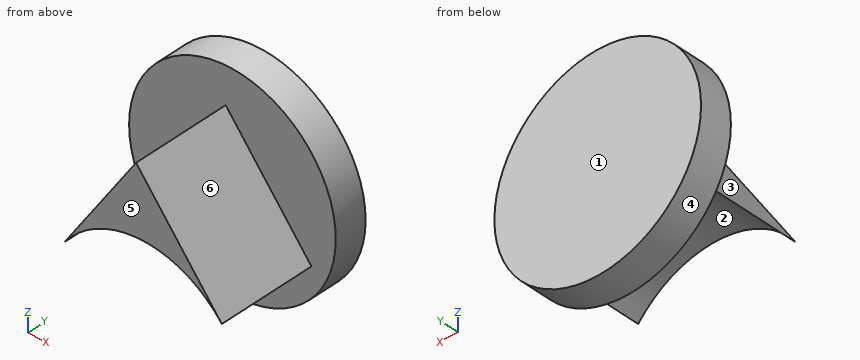
from build123d import *

# Parameters (mm, degrees)
F0_R     = 81.624409
F1_DEPTH = 25.4
F3_DEPTH = 76.2


with BuildPart() as f1:
    # F0 (on Front) → F1 (new body)
    with BuildSketch(Plane.XZ):
        with Locations((-32.545008, 13.374658)):
            Circle(F0_R)
    extrude(amount=F1_DEPTH)

    # F2 (on face) → F3 (join)
    with BuildSketch(Plane.XZ.offset(25.4)):
        with BuildLine():
            Line((-37.894875, 66.024758), (-94.514281, -20.018902))
            ThreePointArc((-94.514281, -20.018902), (-33.306834, 12.514138), (29.870085, -16.006503))
            Line((29.870085, -16.006503), (-37.894875, 66.024758))
        make_face()
    extrude(amount=F3_DEPTH)


solid = f1.part
Input: part model. Units: mm. Frame: model coordinates. Face numbers are marked on the shaded views. A direction names the side the tool comes from. Coordinates: 2 decimals unless noted, no trailing zeros. Loops run counter-clockwise (first coordinate to the right, second up) from the corner with the lowest first, then second, coordinate; pieces in that order, holes last. Notation, with made-up numbers: (9.25, 30.25) - (42.25, 30.25) arc R15 cw to (42.25, 41.25) - close; hole circle Ø10 at (78.25, 68). An arc over 180 degrees is marked (long way). Answer in a Markdown table with one row per item. Add a question column.
Item 1: Section query B-B on z = 10. Return the cut outline in (x, y), then the cut area to 3 significant figures.
Item 2: Contact query for flat-ended pins moving along their axis: P1, Ø8, axis at y = -59, z = -15.5, coming from the -X side; P2, Ø1.5, axis at y = -18, z = 47, coming from the +X side; P3, Ø3, axis at x = 17, z = 39, coming from the +Y side; P4, Ø2, axis at y = -87.5, z = 34.5, coming from the +X side. Output: stop coordinate, or through.
Item 3: Section query A-A on x = -70. Return the cut outline in (y, z).
Item 4: Access query for the marked faces 5 and 6. Directions: +Z, -Z, +X, -X, +Y, -Y. A direction counts if a zero-diameter tool reaches every point of the face in a straight line with its end or side. Return the directions, or none.
Item 5: Line query: line 1 along Y through (x, z) = (-2.5, 86); line 2 along Z through (x, y) = (-31, -12.5); line 3 along X through (y, z) = (-20, 14.5). Output: solid intervals per line, ascending. Write a range as [from, to].
Item 6: Mould query, pull axis X, two halves, no side actions, for the marked faces 1, 2, 3 and 4. Classes: released by +X, released by -X, zero draft, split by the parting line, or undercut.
Item 7: Section query D-D on x = 6.5. Return the cut outline in (y, z).
Item 8: Section query C-C on y = -64.5. Return the cut outline in (x, z), then the cut area to 3 significant figures.
Recorded:
| question | item | result |
|---|---|---|
| 1 | outline | (-114.1, -25.4) - (-74.76, -25.4) - (-74.76, -101.6) - (-50.66, -101.6) - (-50.66, -25.4) - (-10.89, -25.4) - (-10.89, -101.6) - (8.39, -101.6) - (8.39, -25.4) - (49.01, -25.4) - (49.01, 0) - (-114.1, 0) - close |
| 1 | area | 7,450 mm^2 |
| 2 | P1 | x = -94.17 |
| 2 | P2 | x = 42.17 |
| 2 | P3 | y = 0 |
| 2 | P4 | x = -11.03 |
| 3 | outline | (-101.6, 2.07) - (-25.4, 2.07) - (-25.4, -59.15) - (0, -59.15) - (0, 85.9) - (-25.4, 85.9) - (-25.4, 17.24) - (-101.6, 17.24) - close |
| 4 | face 5 | +Z, -Z, +X, -X, -Y |
| 4 | face 6 | +Z, +X, -Y |
| 5 | line 1 | [-25.4, 0] |
| 5 | line 2 | [-68.24, 94.98] |
| 5 | line 3 | [-114.16, 49.07] |
| 6 | face 1 | zero draft |
| 6 | face 2 | undercut |
| 6 | face 3 | released by -X |
| 6 | face 4 | split by the parting line |
| 7 | outline | (-101.6, 3.16) - (-25.4, 3.16) - (-25.4, -58.31) - (0, -58.31) - (0, 85.05) - (-25.4, 85.05) - (-25.4, 12.28) - (-101.6, 12.28) - close |
| 8 | outline | (-94.51, -20.02) arc R78.66 cw to (29.87, -16.01) - (-37.89, 66.02) - close |
| 8 | area | 2,590 mm^2 |
